The model under review builds one solid part; all positions refer to its coordinate system, in mm. A direction names the side the tool comes from. Give positions to 0.01 mm unless a question says otherwise; leave off trailing zeros. Loops run counter-clockwise (first coordinate to the right, second up) from the corner with the lowest first, then second, coordinate; pieces in that order, holes last. Notation, with made-up numbers: (-36, 12.5) -> (-32, 12.5) arc R12 cw to (-32, 25.5) -> close; hole circle Ø11 at (80, -9.75). An arc over 180 degrees is marked (long way). Write each question's results on one line, items separated by ' | '. Start each with the question number.
Q1. Insertion check: pin 1 Ø2 at (x, y) = (8, 2) entering from -Z; pin 2 Ø1.5 at (x, y) = (7, 3) entering from +Z; pin 3 Ø1.5 at (x, y) = (7, 2.5) entering from -Z. Each pin has a flat end and moves straight along its axis. Give the tip position at first contact, or say it passes through.
Q2. We need section B-B (y = 1.25). Write out the cut boundary in (x, z).
Q3. We need section A-A (z = -28). Write out the cut boundary in (x, y), plus the area to 3 significant figures.
Q4. Machinability: for faces 1 (the face through (-5, 3.81, -24)), 2 (the face through (-5, 3, 3.597)), 3 (the face through (7, 3.81, -25)), 4 (the face through (-5, 2.286, -25)), which of the approach directions +Z, -Z, +X, -X, +Y, -Y give a long, thin tool a straight path to every point of the face, cutting with its end or side? Answer none if there is none.
Q5. Wall thickness on L1, parallel to X at y = 1, z = -5; L2, parallel to X at y = 3.75, z = -32.5; L3, parallel to Y at x = -5, z = -19: over which ranges is each line inside the solid? List them lowest first. Write a range as [from, to].
Autodesk Inventor part; units mm, degrees
ref_plane "YZ Plane" through (0, 0, 0) normal (1, 0, 0) x (0, 1, 0)
ref_plane "XZ Plane" through (0, 0, 0) normal (0, 1, 0) x (-1, 0, 0)
ref_plane "XY Plane" through (0, 0, 0) normal (0, 0, 1) x (1, 0, 0)
sketch "Sketch1" plane through (0, 0, 0) normal (0, 1, 0) x (-1, 0, 0)
  line L0 (-6.1647, 4.8669) -> (3.9953, 4.8669)
  line L1 (3.9953, 4.8669) -> (3.9953, -52.2831)
  line L2 (3.9953, -52.2831) -> (-6.1647, -52.2831)
  line L3 (-6.1647, -52.2831) -> (-6.1647, 4.8669)
  point P0 (0, 0)
  dimension "d0" = 10.16
  dimension "d1" = 57.15
extrude "Extrusion1" add sketch "Sketch1" along normal blind 6.096
sketch "Sketch2" plane through (6.1647, 0, 4.8669) normal (1, 0, 0) x (0, 0, -1)
  point P0 (4.8669, 0)
sketch "Sketch3" plane through (6.1647, 0, 4.8669) normal (1, 0, 0) x (0, 0, -1)
  line L0 (0, 0) -> (0, 6.096)
  line L1 (0, 2.286) -> (57.15, 2.286)
  line L2 (57.15, 2.286) -> (57.15, 3.81)
  line L3 (57.15, 3.81) -> (0, 3.81)
  line L4 (0, 3.81) -> (0, 2.286)
  line L5 (57.15, 0) -> (0, 0)
  point P0 (4.8669, 0)
  dimension "d4" = 1.524
  dimension "d5" = 57.15
  dimension "d6" = 2.286
extrude "Extrusion2" add sketch "Sketch3" along normal blind 1.3335
ref_plane "Work Plane1" through (1.0847, 6.096, 4.8669) normal (1, 0, 0) x (0, 0, -1)
mirror "Mirror1" about plane through (1.0847, 6.096, 4.8669) normal (1, 0, 0) of "Extrusion2"
sketch "Sketch4" plane through (6.1647, 0, -52.2831) normal (0, 0, -1) x (-1, 0, 0)
  line L0 (-4.445, 0) -> (14.605, 0)
  line L1 (14.605, 0) -> (14.605, 6.096)
  line L2 (14.605, 6.096) -> (-4.445, 6.096)
  line L3 (-4.445, 6.096) -> (-4.445, 0)
  line L4 (11.4935, 2.286) -> (11.4935, 3.81)
  line L5 (0, 6.096) -> (10.16, 6.096)
  line L6 (5.08, -1.2192) -> (5.08, 7.3152)
  point P0 (6.1647, 0)
  dimension "d12" = 6.096
  dimension "d13" = 19.05
  dimension "d14" = 9.525
extrude "Extrusion3" add sketch "Sketch4" along normal blind 6.35
fillet "Fillet2" radius 6.35 2 edges at (10.6097, 3.048, -58.6331) (-8.4403, 3.048, -58.6331)
sketch "Sketch5" plane through (0, 6.096, 0) normal (0, 1, 0) x (1, 0, 0)
  line L0 (4.2597, 58.6331) -> (-2.0903, 58.6331)
  line L1 (4.2597, 58.6331) -> (4.2597, -15.5891) construction
  line L2 (6.1647, -4.8669) -> (-3.9953, -4.8669)
  arc A0 (4.2597, -4.8669) -> (10.4219, -0.0496) centre (4.2597, 1.4831) ccw
  line L3 (11.5575, 1.4831) -> (7.7347, 1.4831) construction
  line L4 (10.4219, -0.0496) -> (12.4924, -6.8649)
  line L5 (12.4924, -6.8649) -> (5.3123, -7.0975)
  line L6 (5.3123, -7.0975) -> (4.2597, -4.8669)
  point P0 (0, 0)
  dimension "d16" = 6.35
extrude "Extrusion4" cut sketch "Sketch5" against normal blind 7.62
mirror "Mirror2" about plane through (1.0847, 6.096, 4.8669) normal (1, 0, 0) of "Extrusion4"
sketch "Sketch6" plane through (-3.9953, 3.81, -52.2831) normal (-1, 0, 0) x (0, 0, 1)
  line L0 (55.88, 6.0179) -> (62.6058, 6.0179)
  line L1 (62.6058, 6.0179) -> (62.6058, -10.0967)
  line L2 (62.6058, -10.0967) -> (55.88, -10.0967)
  line L3 (55.88, -10.0967) -> (55.88, 6.0179)
  line L4 (0, -3.81) -> (0, 2.286)
  point P0 (52.2831, -3.81)
  dimension "d19" = 55.88
extrude "Extrusion5" cut sketch "Sketch6" along normal blind 7.62
mirror "Mirror3" about plane through (1.0847, 6.096, 4.8669) normal (1, 0, 0) of "Extrusion5"
sketch "Sketch7" plane through (0, 6.096, 0) normal (0, 1, 0) x (1, 0, 0)
  line L0 (-8.4403, 52.2831) -> (10.6097, 52.2831)
  line L1 (10.6097, 52.2831) -> (10.6097, 61.8081)
  line L2 (10.6097, 61.8081) -> (-8.4403, 61.8081)
  line L3 (-8.4403, 61.8081) -> (-8.4403, 52.2831)
  point P0 (0, 0)
  dimension "d22" = 19.05
  dimension "d23" = 9.525
extrude "Extrusion6" add sketch "Sketch7" against normal blind 6.096
fillet "Fillet3" radius 6.35 2 edges at (10.6097, 3.048, -61.8081) (-8.4403, 3.048, -61.8081)
properties part number "Marcus' Case Clip"
Output:
1) pin 1: z = -61.19 | pin 2: z = 3.6 | pin 3: z = -61.49
2) outline: (-8.44, -55.46) arc R6.35 ccw to (-2.09, -61.81) -> (4.26, -61.81) arc R6.35 ccw to (10.61, -55.46) -> (10.61, -52.28) -> (6.16, -52.28) -> (6.16, 4.57) arc R6.35 ccw to (4.26, 4.87) -> (-2.09, 4.87) arc R6.35 ccw to (-4, 4.57) -> (-4, -52.28) -> (-8.44, -52.28) -> close
3) outline: (-5.33, 2.29) -> (-4, 2.29) -> (-4, 0) -> (6.16, 0) -> (6.16, 2.29) -> (7.5, 2.29) -> (7.5, 3.81) -> (6.16, 3.81) -> (6.16, 6.1) -> (-4, 6.1) -> (-4, 3.81) -> (-5.33, 3.81) -> close | area: 66.0 mm2
4) face 1: +Z, -X, +Y | face 2: +Z, -X, +Y, -Y | face 3: +Z, +X, +Y | face 4: +Z, -X, -Y
5) L1: [-4, 6.16] | L2: [-5.33, 7.5] | L3: [2.29, 3.81]
